```python
from build123d import *

# Parameters (mm, degrees)
F0_R          = 1.6764
F1_DEPTH      = 4.826
F2_R          = 1.6764
F3_DEPTH      = 4.826
F3_DEPTH_BACK = 9.652


with BuildPart() as f1:
    # F0 (on Front) → F1 (new body)
    with BuildSketch(Plane.XZ):
        with BuildLine():
            Line((0, 25.4), (0, 0))
            Line((0, 0), (12.7, 0))
            Line((12.7, 0), (12.7, 12.7))
            Line((12.7, 12.7), (63.5, 12.7))
            Line((63.5, 12.7), (63.5, 6.35))
            Line((63.5, 6.35), (73.025, 6.35))
            ThreePointArc((73.025, 6.35), (75.2700640303, 7.2799359697), (76.2, 9.525))
            Line((76.2, 9.525), (76.2, 25.4))
            Line((76.2, 25.4), (0, 25.4))
        make_face()
        with BuildLine():
            add(Edge.make_bspline(
                [(76.2, 25.4), (26.6581273418, 36.622909108), (-29.7852053598, 44.2043974935), (-20.7405121115, 0), (0, 0)],
                knots=[0, 0, 0, 0, 0.6344075171, 1, 1, 1, 1], degree=3))
            Line((0, 0), (0, 25.4))
            Line((0, 25.4), (76.2, 25.4))
        make_face()
        with Locations((-6.35, 15.875)):
            Circle(F0_R, mode=Mode.SUBTRACT)
        with Locations((6.35, 31.115)):
            Circle(F0_R, mode=Mode.SUBTRACT)
    extrude(amount=F1_DEPTH)

    # F2 (on face) → F3 (join, two sides)
    with BuildSketch(Plane.XZ.offset(4.826)) as f3_sk:
        with BuildLine():
            Line((3.175, 27.3878005167), (19.7676480954, 27.3878005167))
            Line((19.7676480954, 27.3878005167), (25.0090726158, 34.7748551155))
            add(Edge.make_bspline(
                [(25.0090726158, 34.7748551155), (2.6249492009, 37.1897339417), (-27.5347979466, 33.2059146169), (-20.7405121115, 0), (0, 0)],
                knots=[0.2488096999, 0.2488096999, 0.2488096999, 0.2488096999, 0.6344075171, 1, 1, 1, 1], degree=3))
            Line((0, 0), (0, 24.2128005167))
            ThreePointArc((0, 24.2128005167), (0.9299359697, 26.457864547), (3.175, 27.3878005167))
        make_face()
        with Locations((-6.35, 15.875)):
            Circle(F2_R, mode=Mode.SUBTRACT)
        with Locations((6.35, 31.115)):
            Circle(F2_R, mode=Mode.SUBTRACT)
    extrude(amount=F3_DEPTH)
    extrude(f3_sk.sketch, amount=-F3_DEPTH_BACK)


solid = f1.part
```
The listing builds one solid part. Answer for the finished solid, in the listing's coordinates (mm). A direction names the side the tool comes from. Give positions to 0.01 mm unless a question says otherwise; leave off trailing zeros. Return JSON: item names as keys, results as strings. Group by question number.
1. Find section A-A (y = 1.5). State how many separate pieces and enclosed holes the cut face has, then the cut area to 3 significant figures.
2. Determine the mould class of faces 1 (the flat face through (22.35, -7.21, 31.03)), 2 (the flat face through (68, -2, 6.35)), 3 (the flat face through (38, -2, 12.7)) for opening direction X: pulls with the +X half, pulls with the -X half, needs draft (parallel to the pull), parting line crosses it, or undercut.
3. Which of the six approach directions +Z, -Z, +X, -X, +Y, -Y give full straight-line access (tool end or side, diameter ignored) to faces 4 (the flat face through (11, -7, 27.388)), 5 (the flat face through (12.7, -2, 6)), 6 (the flat face through (6, -2, 0)), 7 (the flat face through (11, 2, 27.388))?
4. Given pin 1 Ø1.4 at (y, z) = (-1.5, 7.5) entering from +X; pin 2 Ø2.5 at (y, z) = (3, 10) entering from +X; pin 3 Ø2.5 at (x, y) = (11, -7.5) entering from -Z, each flat-ended and moving along its own axis, determine where each tip first touches the part or whether it passes through.
5. Straight lines are drawn through the part: line 1 (Z direction, x = 25, y = -0.5); line 2 (Z direction, x = 6.35, y = 2.65); line 3 (X direction, y = -8, z = 14.5). For each, find the intervals that lie inside material, in ascending order. Write a range as [from, to].
Verdict:
{
 "1": {"separate pieces": "1", "enclosed holes": "2", "area": "750 mm^2"},
 "2": {"face 1": "pulls with the +X half", "face 2": "needs draft", "face 3": "undercut"},
 "3": {"face 4": "-Z, +X, -Y", "face 5": "-Z, +Y, -Y", "face 6": "-Z, +X, -X, +Y, -Y", "face 7": "-Z, +X, +Y"},
 "4": {"pin 1": "stops at x = 75.91", "pin 2": "stops at x = 0", "pin 3": "stops at z = 27.39"},
 "5": {"line 1": "z = [12.7, 34.78]", "line 2": "z = [27.39, 29.44], [32.79, 35.64]", "line 3": "x = [-20.78, -7.31], [-5.39, 0]"}
}
